```python
from build123d import *

# Parameters (mm, degrees)
SKETCH4_W           = 28
SKETCH4_H           = 45
BOSS_EXTRUDE2_DEPTH = 10
SKETCH6_R           = 2.15
CUT_EXTRUDE1_DEPTH  = 6
SKETCH7_R           = 2.75
CUT_EXTRUDE2_DEPTH  = 6


with BuildPart() as part:
    # Sketch4 → Boss-Extrude2 (new body)
    with BuildSketch(Plane.XY):
        Rectangle(SKETCH4_W, SKETCH4_H)
    extrude(amount=BOSS_EXTRUDE2_DEPTH)

    # Sketch5 → Cut-Revolve1 (revolve, cut)
    with BuildSketch(Plane.XY.offset(10)):
        Polygon((0, 22.5), (8.33, 22.5), (8.33, 16.5), (6, 10.5), (4.75, -18.71), (4.75, -22.5), (0, -22.5), align=None)
    revolve(axis=Axis((0, 0, 10), (0, 1, 0)), mode=Mode.SUBTRACT)

    # Sketch6 → Cut-Extrude1 (cut)
    with BuildSketch(Plane.XY.offset(10)):
        with Locations((-10.5, 6.5)):
            Circle(SKETCH6_R)
        with Locations((-10.5, -17.5)):
            Circle(SKETCH6_R)
        with Locations((10.5, 6.5)):
            Circle(SKETCH6_R)
        with Locations((10.5, -17.5)):
            Circle(SKETCH6_R)
    extrude(amount=-CUT_EXTRUDE1_DEPTH, mode=Mode.SUBTRACT)

    # Sketch7 → Cut-Extrude2 (cut)
    with BuildSketch(Plane(origin=(0, 0, 0), x_dir=(-1, 0, 0), z_dir=(0, 0, -1))):
        with Locations((-10, 12.5)):
            Circle(SKETCH7_R)
        with Locations((10, 12.5)):
            Circle(SKETCH7_R)
    extrude(amount=-CUT_EXTRUDE2_DEPTH, mode=Mode.SUBTRACT)


solid = part.part
```
Read the model definition and answer for the solid it produces. Units are mm, in the model's axes. A direction names the side the tool comes from. Round coordinates to 2 decimals unless told otherwise and drop trailing zeros. Write each loop counter-clockwise with the first axis right and the second up, starting at its lowest first coordinate (ties: lowest second). Pieces come first, ordered by that corner, then holes. Notation, with made-up numbers: (67, -32) - (74, -32) arc R13 ccw to (74, -26) - close; hole circle Ø3 at (52.25, 77.5). An arc over 180 degrees is marked (long way). Use CSV: the item, a comma, the result in double quotes.
Q1. Each of these flat-tipped pins is pushed along its axis until it touches: pin 1 Ø1.3 at (x, y) = (-10, -18) entering from +Z; pin 2 Ø3 at (x, y) = (-2, 15.5) entering from +Z; pin 3 Ø5 at (x, y) = (-10, 12.5) entering from -Z. Where does it stop, or does it pass through?
Values:
pin 1,"stops at z = 4"
pin 2,"stops at z = 3.12"
pin 3,"stops at z = 6"
Q2. Find section D-D, the plane x = 10. Write down the section's boundary in (y, z), then the cut area to 3 significant figures.
Values:
outline,"(-22.5, 0) - (9.75, 0) - (9.75, 6) - (15.25, 6) - (15.25, 0) - (22.5, 0) - (22.5, 10) - (8.59, 10) - (8.59, 4) - (4.41, 4) - (4.41, 10) - (-15.41, 10) - (-15.41, 4) - (-19.59, 4) - (-19.59, 10) - (-22.5, 10) - close"
area,"367 mm²"
Q3. Determine the mould class of faces 1 (the conical face through (0.118, -4.309, 4.635)), 2 (the flat face through (9, 0, 10)), 3 (the flat face through (-10, 13, 6)) for opening direction Y: +Y half, -Y half, draft (parallel to the pull), parting line (faces both ways), or undercut.
Values:
face 1,"+Y half"
face 2,"draft"
face 3,"undercut"
Q4. Straight lines are drawn through the part: line 1 along Y through (x, z) = (10.5, 6.2); line 2 along Y through (x, z) = (-8.75, 8.75); line 3 along X through (y, z) = (-16, 8.75). For each, find the intervals that lie inside material, in ascending order.
Values:
line 1,"y = -22.5 to -19.65, -15.35 to 4.35, 8.65 to 22.5"
line 2,"y = -22.5 to -18.75, -16.25 to 5.25, 7.75 to 22.5"
line 3,"x = -14 to -12.04, -8.96 to -4.7, 4.7 to 8.96, 12.04 to 14"
Q5. Find section B-B, the plane y = -17.5. Write down the section's boundary in (x, z), then the cut area to 3 significant figures.
Values:
outline,"(-14, 0) - (14, 0) - (14, 10) - (12.65, 10) - (12.65, 4) - (8.35, 4) - (8.35, 10) - (4.8, 10) arc R4.8 cw to (-4.8, 10) - (-8.35, 10) - (-8.35, 4) - (-12.65, 4) - (-12.65, 10) - (-14, 10) - close"
area,"192 mm²"
Q6. Find section A-A, the plane x = 0. Write down the section's boundary in (y, z), then the cut area to 3 significant figures.
Values:
outline,"(-22.5, 0) - (22.5, 0) - (22.5, 1.67) - (16.5, 1.67) - (10.5, 4) - (-18.71, 5.25) - (-22.5, 5.25) - close"
area,"182 mm²"
Q7. A tool of negligible diameter and unlimited length cuts with its end or side. For faces 4 (the cylindrical face through (-12.62, 13.33, 2.96)), 5 (the flat face through (-0.2, 22.5, 0.5)), 6 (the cylindrical face through (10.22, 8.63, 7.04)), from which of +Z, -Z, +X, -X, +Y, -Y can it reach the whole face along a straight path? Write none if from no direction.
Values:
face 4,"-Z"
face 5,"+Z, -Z, +X, -X, +Y"
face 6,"+Z"
Q8. Find section C-C, the plane z = 2.75. Count the separate pieces of the cut face and the enclosed holes in it, then the cut area to 3 significant figures.
Values:
separate pieces,"1"
enclosed holes,"2"
area,"1,150 mm²"
